Source: CAD feature listing. Evaluate the final solid. Frame: model axes, mm. Round coordinates to 2 decimals unless told otherwise and drop trailing zeros. Order: outer loops, then holes, each group sorted by start corner. A loop starts at its lowest first (then second) coordinate and runs counter-clockwise, first axis right, second up. Notation, with made-up numbers: M 7,-3 L 56,-3 A36 ccw 56,32 Z; hole C 77.5,-38 d7. An arc over 180 degrees is marked long. Use one line per item in the form item = value. Start each with the question number.
Q1. Section B-B (y = 79). Return the cut outline in (x, z).
Q2. Contact query for flat-ended pins moving along their axis: pin 1 (1 mm diameter, centred on x = 106.56, y = 56, fed in from -Z); pin 2 (2 mm diameter, centred on x = -1.5, z = 0.5, fed in from +Y). Output: stop coordinate, or through.
Q3. Section A-A (z = 3.35). Give the number of separate pieces and of enclosed holes in the cut face, plus the area to 3 significant figures.
Q4. Material intervals for probe 1 along X at (y, z) = (105.5, 1.75); probe 2 along Y at (x, z) = (93.5, 0.25); probe 3 along X at (y, z) = (28, 2.65), sorted ascending.
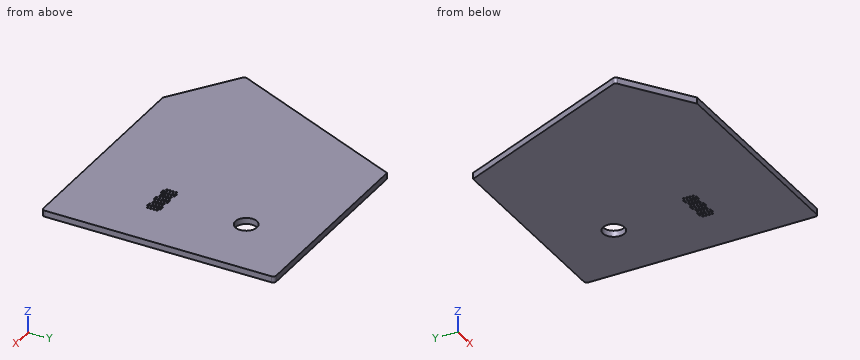
from build123d import *

# Parameters (mm, degrees)
RESSALTO_EXTRUS_O1_DEPTH                 = 4
ESBO_O2_R                                = 0.5
CORTE_EXTRUS_O1_DEPTH                    = 206.554088373
ESBO_O2_7_R                              = 0.5
CORTE_EXTRUS_O2_DEPTH                    = 206.554088373
ESBO_O2_9_R                              = 7
CORTE_EXTRUS_O3_DEPTH                    = 206.554088373
ESBO_O2_10_R                             = 0.5
CORTE_EXTRUS_O4_DEPTH                    = 206.554088373
ESBO_O2_11_R                             = 0.5
CORTE_EXTRUS_O5_DEPTH                    = 206.554088373
FURO_DE_DI_METRO_1_15_1_15_1_D           = 1.15
FURO_DE_DI_METRO_1_15_1_15_1_CSINK_D     = 1.2
FURO_DE_DI_METRO_1_15_1_15_1_CSINK_ANGLE = 90
FURO_DE_DI_METRO_1_0_1_1_D               = 1
FURO_DE_DI_METRO_1_0_1_1_CSINK_D         = 1.05
FURO_DE_DI_METRO_1_0_1_1_CSINK_ANGLE     = 90


with BuildPart() as part:
    # Esboço1 → Ressalto-extrusão1 (new body)
    with BuildSketch(Plane.XY):
        with BuildLine():
            Line((0, 0), (138, 0))
            ThreePointArc((138, 0), (139.414213562, 0.585786438), (140, 2))
            Line((140, 2), (140, 148.454256327))
            ThreePointArc((140, 148.454256327), (139.414213562, 149.86846989), (138, 150.454256327))
            Line((138, 150.454256327), (9.899407771, 150.454256327))
            Line((9.899407771, 150.454256327), (-41.646512669, 31.110140067))
            ThreePointArc((-41.646512669, 31.110140067), (-41.734695124, 29.77189369), (-40.957602214, 28.678821818))
            Line((-40.957602214, 28.678821818), (0, 0))
        make_face()
    extrude(amount=RESSALTO_EXTRUS_O1_DEPTH)

    # Esboço2 → Corte-extrusão1 (cut, through all)
    with BuildSketch(Plane.XY.offset(4)):
        with Locations((104.555415111, 50)):
            Circle(ESBO_O2_R)
    extrude(amount=-CORTE_EXTRUS_O1_DEPTH, mode=Mode.SUBTRACT)

    # Esboço2<7> → Corte-extrusão2 (cut, through all)
    with BuildSketch(Plane.XY.offset(4)):
        with Locations((100.555415111, 57)):
            Circle(ESBO_O2_7_R)
    extrude(amount=-CORTE_EXTRUS_O2_DEPTH, mode=Mode.SUBTRACT)

    # Esboço2<9> → Corte-extrusão3 (cut, through all)
    with BuildSketch(Plane.XY.offset(4)):
        with Locations((97.555415111, 108.436764235)):
            Circle(ESBO_O2_9_R)
    extrude(amount=-CORTE_EXTRUS_O3_DEPTH, mode=Mode.SUBTRACT)

    # Esboço2<10> → Corte-extrusão4 (cut, through all)
    with BuildSketch(Plane.XY.offset(4)):
        with Locations((88.555415111, 58)):
            Circle(ESBO_O2_10_R)
    extrude(amount=-CORTE_EXTRUS_O4_DEPTH, mode=Mode.SUBTRACT)

    # Esboço2<11> → Corte-extrusão5 (cut, through all)
    with BuildSketch(Plane.XY.offset(4)):
        with Locations((90.555415111, 58)):
            Circle(ESBO_O2_11_R)
    extrude(amount=-CORTE_EXTRUS_O5_DEPTH, mode=Mode.SUBTRACT)

    # Furo de diâmetro Ø1.15 (1.15)1 (through all)
    with Locations(Plane(origin=(106.555415111, 56, 4), x_dir=(1, 0, 0), z_dir=(0, 0, 1))):
        with Locations((0, 0), (2, 1), (2, -1), (2, -3)):
            CounterSinkHole(FURO_DE_DI_METRO_1_15_1_15_1_D / 2, FURO_DE_DI_METRO_1_15_1_15_1_CSINK_D / 2, counter_sink_angle=FURO_DE_DI_METRO_1_15_1_15_1_CSINK_ANGLE)

    # Furo de diâmetro Ø1.0 (1)1 (through all)
    with Locations(Plane(origin=(106.555415111, 58, 4), x_dir=(1, 0, 0), z_dir=(0, 0, 1))):
        with Locations((0, 0), (-2, 0), (-4, -1), (-6, -1), (-4, -3), (-2, -2), (-2, -4), (0, -4), (0, -6), (2, -7), (0, -8), (-2, -6), (-14, -1), (-14, -3), (-14, -5), (-14, -7), (-12, -7), (-10, -8), (-8, -8), (-6, -7), (-4, -7), (-4, -5), (-6, -5), (-6, -3), (-8, -2), (-8, 0), (-10, 0), (-10, -2), (-10, -4), (-8, -4), (-10, -6), (-8, -6), (-12, -5), (-12, -3), (-12, -1), (-18, 0), (-16, 0), (-20, -1), (-18, -2), (-16, -2), (-16, -4), (-16, -6), (-16, -8), (-18, -8), (-18, -6), (-18, -4), (-20, -3), (-20, -5), (-20, -7)):
            CounterSinkHole(FURO_DE_DI_METRO_1_0_1_1_D / 2, FURO_DE_DI_METRO_1_0_1_1_CSINK_D / 2, counter_sink_angle=FURO_DE_DI_METRO_1_0_1_1_CSINK_ANGLE)


solid = part.part
Results list:
q1.outline = M -20.96,0 L 140,0 L 140,4 L -20.96,4 Z
q2.pin_1 = through
q2.pin_2 = 126.38
q3.separate_pieces = 1
q3.enclosed_holes = 55
q3.area = 23,400 mm2
q4.probe_1 = -9.52 to 91.2, 103.91 to 140
q4.probe_2 = 0 to 102.73, 114.14 to 150.45
q4.probe_3 = -39.99 to 140
